Work out the finished part from the listing and answer in its coordinate system (mm). Face numbers are marked on the shaded views. Coordinates: 2 decimals unless noted, no trailing zeros. Order: outer loops, then holes, each group sorted by start corner. A loop starts at its lowest first (then second) coordinate and runs counter-clockwise, first axis right, second up. Notation, with made-up numbers: M 20,-19.75 L 25,-19.75 A18 cw 25,-11.75 Z; hole C 62,16.25 d2. An arc over 180 degrees is marked long. Write item = value, one per line. Start each with the question number.
Q1. Find section B-B on y = 0. Give the vertices of the cut face in (x, z), and give its area (3 significant figures).
Q2. Determine the mould class of the marked faces 1, 2 and 3 for opening direction Y: released by +Y, released by -Y, zero draft, split by the parting line, or undercut.
Q3. Find section D-D on x = -13.5. Give the vertices of the cut face in (y, z), and give its area (3 significant figures).
Q4. Straight lines are drawn through the part: line 1 along Y through (x, z) = (0, -2.85); line 2 along Y through (x, z) = (33, -3.3); line 3 along Y through (x, z) = (-31, -1.7). For each, find the intervals that lie inside material, in ascending order.
Q5. Each of these flat-tipped pins is pushed along its axis until it touches: P1, Ø3, axis at x = 40.5, y = 24, coming from the +Z side; P2, Ø1, axis at y = 37, z = -1, coming from the +X side; P3, Ø0.8, axis at x = 0, y = -47, coming from the +Z side; P4, Ø4, axis at x = -35, y = 19, coming from the +Z side. Where does it stop, or does it pass through?
Q6. Find section C-C on z = -3.9. Give the vertices of the cut face in (x, y).
Q7. Find section A-A on x = 0. Give the vertices of the cut face in (y, z).
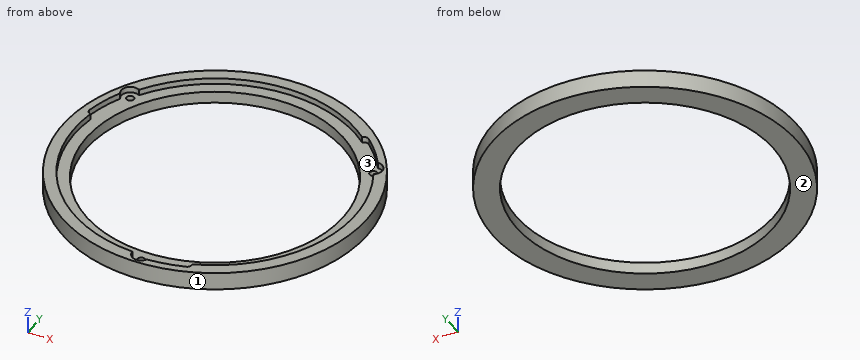
Autodesk Fusion 360 part; units mm, degrees
sketch "草图1" plane through (0, 0, 0) normal (0, 0, 1) x (1, 0, 0)
  line L0 (0.9, -43.0906) -> (0.9, -43.1)
  arc A0 (2.5554, -45.5283) -> (2.6381, -48.5283) centre (0, -47.1) ccw
  line L1 (28.4627, -32.3648) -> (28.4702, -32.3737)
  arc A1 (14.7507, -46.3074) -> (13.8402, -43.4489) centre (14.2954, -44.8782) ccw
  line L2 (30.5781, -30.3742) -> (30.6917, -30.5096)
  arc A2 (2.6381, -48.5283) -> (14.7507, -46.3074) centre (0, 0) ccw
  line L3 (42.2601, -8.467) -> (42.2716, -8.469)
  circle A3 centre (0, 0) radius 43.1
  line L4 (11.0158, 41.6685) -> (11.0763, 41.8346)
  arc A4 (-47.4788, 10.3792) -> (-44.548, 9.7385) centre (-46.0134, 10.0589) ccw
  circle A5 centre (40.7898, 23.55) radius 1.25
  line L5 (-11.0158, 41.6685) -> (-11.0763, 41.8346)
  line L6 (-36.8676, 22.3247) -> (-36.8757, 22.3294)
  line L7 (36.8676, 22.3247) -> (36.8757, 22.3294)
  line L8 (-13.7974, 40.8319) -> (-13.8014, 40.8428)
  circle A6 centre (0, 0) radius 47.1 construction
  line L9 (41.5939, -11.2943) -> (41.768, -11.325)
  arc A7 (38.151, 24.9772) -> (30.7078, 33.7104) centre (0, 0) ccw
  arc A8 (-43.3459, 21.9795) -> (-47.4788, 10.3792) centre (0, 0) ccw
  line L10 (-41.5939, -11.2943) -> (-41.768, -11.325)
  line L11 (-28.4627, -32.3648) -> (-28.4702, -32.3737)
  line L12 (-37.7676, 20.7659) -> (-37.7757, 20.7706)
  arc A9 (32.728, 35.9282) -> (30.7078, 33.7104) centre (31.7179, 34.8193) ccw
  arc A10 (-40.7064, 20.5512) -> (-44.548, 9.7385) centre (0, 0) ccw
  circle A11 centre (0, 0) radius 44.72 construction
  arc A12 (40.7077, 26.5489) -> (32.728, 35.9282) centre (0, 0) ccw
  line L13 (-0.9, -43.0906) -> (-0.9, -43.1)
  arc A13 (-40.7064, 20.5512) -> (-43.3459, 21.9795) centre (-40.7898, 23.55) ccw
  arc A14 (38.151, 24.9772) -> (40.7077, 26.5489) centre (40.7898, 23.55) ccw
  circle A15 centre (0, 0) radius 51.1
  line L14 (13.7974, 40.8319) -> (13.8014, 40.8428)
  circle A16 centre (0, -47.1) radius 1.25
  line L15 (-30.5781, -30.3742) -> (-30.6917, -30.5096)
  line L16 (-42.2601, -8.467) -> (-42.2716, -8.469)
  arc A17 (2.5554, -45.5283) -> (13.8402, -43.4489) centre (0, 0) ccw
  circle A18 centre (-40.7898, 23.55) radius 1.25
  line L17 (37.7676, 20.7659) -> (37.7757, 20.7706)
  line L18 (-15.6751, 9.05) -> (-16.3679, 9.45) construction
  line L19 (-37.3257, 21.55) -> (-41.5692, 24) construction
  line L20 (43.1, 0) -> (48, 0) construction
  line L21 (0, -43.1) -> (0, -51.1) construction
  circle A19 centre (0, 0) radius 47.1
  dimension "d17" = 1.8
  dimension "d22" = 6
  dimension "d23" = 3
  dimension "d24" = 2.5
  dimension "d25" = 2.5
  dimension "d26" = 2.5
  dimension "d27" = 86.2
  dimension "d28" = 102.2
extrude "拉伸4" add sketch "草图1" against normal blind 6 contours A0 A1 A16 A17 A19 | A0 A1 A4 A7 A9 A10 A13 A14 A17 A19 | A0 A1 A2 A16 A19 | A4 A10 A13 A18 A19 | A4 A8 A13 A18 A19 | A16 A19 | A16 A19 | A18 A19 | A18 A19 | A5 A9 A12 A14 A19 | A5 A7 A9 A14 A19 | A5 A19 | A5 A19 | A15
extrude "拉伸5" cut sketch "草图1" against normal blind 2 contours A0 A1 A16 A17 A19 | A0 A1 A4 A7 A9 A10 A13 A14 A17 A19 | A0 A1 A2 A16 A19 | A4 A10 A13 A18 A19 | A4 A8 A13 A18 A19 | A16 A19 | A16 A19 | A18 A19 | A18 A19 | A5 A9 A12 A14 A19 | A5 A7 A9 A14 A19 | A5 A19 | A5 A19
extrude "拉伸6" cut sketch "草图1" against normal blind 5 contours A16 A19 | A16 A19 | A18 A19 | A18 A19 | A5 A19 | A5 A19
Findings below:
q1.outline = M -51.1,-6 L -43.1,-6 L -43.1,-2 L -47.1,-2 L -47.1,0 L -51.1,0 Z; M 43.1,-6 L 51.1,-6 L 51.1,0 L 47.1,0 L 47.1,-2 L 43.1,-2 Z
q1.area = 80.0 mm^2
q2.face_1 = split by the parting line
q2.face_2 = zero draft
q2.face_3 = undercut
q3.outline = M -49.28,-6 L -40.93,-6 L -40.93,-2 L -45.12,-2 L -45.12,0 L -49.28,0 Z; M 40.93,-6 L 49.28,-6 L 49.28,0 L 45.12,0 L 45.12,-2 L 40.93,-2 Z
q3.area = 83.5 mm^2
q4.line_1 = -51.1 to -48.35, -45.85 to -43.1, 43.1 to 51.1
q4.line_2 = -39.02 to -27.72, 27.72 to 39.02
q4.line_3 = -40.62 to -35.46, 35.46 to 40.62
q5.P1 = -2
q5.P2 = 35.76
q5.P3 = -5
q5.P4 = through
q6.outline = C 0,0 d102.2; hole C 0,0 d86.2; hole C -40.79,23.55 d2.5; hole C 0,-47.1 d2.5; hole C 40.79,23.55 d2.5
q7.outline = M -51.1,-6 L -43.1,-6 L -43.1,-2 L -45.85,-2 L -45.85,-5 L -48.35,-5 L -48.35,-2 L -50.1,-2 L -50.1,0 L -51.1,0 Z; M 43.1,-6 L 51.1,-6 L 51.1,0 L 47.1,0 L 47.1,-2 L 43.1,-2 Z
